Input: part model. Units: mm. Frame: model coordinates. A direction names the side the tool comes from. Coordinates: 2 decimals unless noted, no trailing zeros. Order: outer loops, then holes, each group sorted by start corner. A loop starts at its lowest first (then second) coordinate and runs counter-clockwise, first axis right, second up. Notation, with made-up numbers: (62, 69) -> (108, 69) arc R22 cw to (108, 93) -> close; hole circle Ø4 at (-0.75, 23). An arc over 180 degrees is marked (long way). Use one line per item in the form item = value. Start each with the question number.
1) Draft query along Y for faces 1 (the flat face through (0, -3, 0)), 2 (the flat face through (-8, -8.7, 3)), 3 (the cylindrical face through (-1.72, -1.99, 2.54)). Return one class per face: pulls with the +Y half, pulls with the -Y half, needs draft (parallel to the pull), parting line crosses it, or undercut.
2) Section query C-C on y = 3.5. Output: boundary loops of the cut face in (x, z), then the cut area to 3 significant figures.
3) Pin query (flat end, axial travel): pin 1 (1.3 mm diameter, centred on y = -11.5, z = 3.5, fed in from -X); pin 2 (1 mm diameter, centred on x = -10.5, z = 4.5, fed in from +Y); pin 3 (2 mm diameter, centred on y = -11.5, z = 2, fed in from +X). Return the tip coordinate at first contact, or that it passes through.
4) Ray query, line 1 along X through (y, z) = (6, 3.25) (3 decimals); line 2 along X through (y, z) = (-9.5, 2.75); line 3 along Y through (x, z) = (0, 2.4) (3 decimals). Return the intervals inside material, ascending.
5) Section query B-B on z = 3.7. Output: boundary loops of the cut face in (x, y) (3 decimals).
6) Section query D-D on x = 0. Output: boundary loops of the cut face in (y, z) (3 decimals).
7) Section query A-A on y = 6.75. Output: boundary loops of the cut face in (x, z).
8) Access query for faces 4 (the cylindrical face through (8.035, 7.506, 2.535)), 5 (the flat face through (-10, 11.03, 2.54)), 6 (the flat face through (3, -11, 3)), 7 (the flat face through (-3, -11, 3)). Directions: +Z, -Z, +X, -X, +Y, -Y. A direction counts if a zero-diameter tool reaches every point of the face in a straight line with its end or side. Return the directions, or none.
from build123d import *

# Parameters (mm, degrees)
F0_W     = 26
F0_H     = 26
F1_DEPTH = 5
F3_DEPTH = 25
F4_W     = 10
F4_H     = 4.3
F5_DEPTH = 25


with BuildPart() as f1:
    # F0 (on Top) → F1 (new body)
    with BuildSketch(Plane.XY):
        Rectangle(F0_W, F0_H)
    extrude(amount=F1_DEPTH)

    # F2 (on face) → F3 (cut)
    with BuildSketch(Plane.XY.offset(5)):
        with BuildLine():
            ThreePointArc((-7.604645, 9), (-1.526868, -2.031146), (8.175, 6))
            ThreePointArc((8.175, 6), (8.031146, 7.526868), (7.604645, 9))
            ThreePointArc((7.604645, 9), (6.242686, 11.27821), (4.222632, 13))
            Line((4.222632, 13), (-4.222632, 13))
            ThreePointArc((-4.222632, 13), (-6.242686, 11.27821), (-7.604645, 9))
        make_face()
        with BuildLine():
            ThreePointArc((4.222632, 13), (6.242686, 11.27821), (7.604645, 9))
            Line((7.604645, 9), (12.328957, 13))
            Line((12.328957, 13), (4.222632, 13))
        make_face()
        with BuildLine():
            Line((-12.328957, 13), (-7.604645, 9))
            ThreePointArc((-7.604645, 9), (-6.242686, 11.27821), (-4.222632, 13))
            Line((-4.222632, 13), (-12.328957, 13))
        make_face()
        with BuildLine():
            Line((-4.222632, 13), (4.222632, 13))
            ThreePointArc((4.222632, 13), (0, 14.175), (-4.222632, 13))
        make_face()
    extrude(amount=-F3_DEPTH, mode=Mode.SUBTRACT)

    # F4 (on face) → F5 (cut)
    with BuildSketch(Plane.XY.offset(5)):
        with Locations((-8, -10.85)):
            Rectangle(F4_W, F4_H)
        with Locations((8, -10.85)):
            Rectangle(F4_W, F4_H)
    extrude(amount=-F5_DEPTH, mode=Mode.SUBTRACT)


solid = f1.part
Answers below:
q1.face_1 = needs draft
q1.face_2 = pulls with the -Y half
q1.face_3 = undercut
q2.outline = (-13, 0) -> (-7.78, 0) -> (-7.78, 5) -> (-13, 5) -> close; (7.78, 0) -> (13, 0) -> (13, 5) -> (7.78, 5) -> close
q2.area = 52.2 mm^2
q3.pin_1 = -3
q3.pin_2 = 11.87
q3.pin_3 = 3
q4.line_1 = -13 to -8.175, 8.175 to 13
q4.line_2 = -3 to 3
q4.line_3 = -13 to -2.175
q5.outline = (-13, -8.7) -> (-3, -8.7) -> (-3, -13) -> (3, -13) -> (3, -8.7) -> (13, -8.7) -> (13, 13) -> (12.329, 13) -> (7.605, 9) arc R8.175 cw to (8.175, 6) arc R8.175 cw (long way) to (-7.605, 9) -> (-12.329, 13) -> (-13, 13) -> close
q6.outline = (-13, 0) -> (-2.175, 0) -> (-2.175, 5) -> (-13, 5) -> close
q7.outline = (-13, 0) -> (-8.14, 0) -> (-8.14, 5) -> (-13, 5) -> close; (8.14, 0) -> (13, 0) -> (13, 5) -> (8.14, 5) -> close
q8.face_4 = +Z, -Z
q8.face_5 = +Z, -Z, +Y
q8.face_6 = +Z, -Z, +X, -Y
q8.face_7 = +Z, -Z, -X, -Y
